```python
from build123d import *

# Parameters (mm, degrees)
SKETCH218_R     = 1.8
SKETCH218_R_2   = 1.5
PAD127054_DEPTH = 3
PAD127055_DEPTH = 2.5


with BuildPart() as base:
    # Sketch218 → Pad127054 (new body)
    with BuildSketch(Plane(origin=(50, 160, 11.5), x_dir=(1, 0, 0), z_dir=(0, 0, 1))):
        with BuildLine():
            Line((-40, 8.5), (-40, 10.5))
            Line((-40, 10.5), (-43, 10.5))
            Line((-43, 10.5), (-44.5, 10.5))
            Line((-44.5, 10.5), (-44.5, 7.5))
            Line((-44.5, 7.5), (-47.5, 7.5))
            Line((-47.5, 7.5), (-47.5, 10.5))
            Line((-47.5, 10.5), (-50, 10.5))
            Line((-50, -67), (-50, 10.5))
            Line((-28, -67), (-50, -67))
            Line((-24.376533, -53.477038), (-28, -67))
            Line((-29.344931, -44.194174), (-24.376533, -53.477038))
            Line((-22.98097, -37.830213), (-29.344931, -44.194174))
            Line((-22.98097, -37.830213), (-20.85965, -35.708892))
            Line((-20.85965, -35.708892), (-22.273864, -34.294679))
            Line((-17.847446, -29.868261), (-22.273864, -34.294679))
            Line((-24, -15.512303), (-17.847446, -29.868261))
            Line((-24, 0), (-24, -15.512303))
            ThreePointArc((-24, 0), (-24.87868, 2.12132), (-27, 3))
            Line((-37.721825, 3), (-27, 3))
            Line((-40, 8.5), (-37.721825, 3))
        make_face()
        with Locations((-27, 0)):
            Circle(SKETCH218_R, mode=Mode.SUBTRACT)
        with Locations((-27, -10)):
            Circle(SKETCH218_R, mode=Mode.SUBTRACT)
        with Locations((-23, -28)):
            Circle(SKETCH218_R, mode=Mode.SUBTRACT)
        with Locations((-35, 0)):
            Circle(SKETCH218_R, mode=Mode.SUBTRACT)
        with Locations((-32, -63)):
            Circle(SKETCH218_R_2, mode=Mode.SUBTRACT)
        with Locations((-42, -63)):
            Circle(SKETCH218_R_2, mode=Mode.SUBTRACT)
        with Locations((-32, -56)):
            Circle(SKETCH218_R_2, mode=Mode.SUBTRACT)
        with Locations((-42, -56)):
            Circle(SKETCH218_R_2, mode=Mode.SUBTRACT)
        with Locations((-44.4, -49)):
            Circle(SKETCH218_R, mode=Mode.SUBTRACT)
        with Locations((-44.4, -41)):
            Circle(SKETCH218_R, mode=Mode.SUBTRACT)
        with Locations((-44.4, -11)):
            Circle(SKETCH218_R, mode=Mode.SUBTRACT)
        with Locations((-44.4, -3)):
            Circle(SKETCH218_R, mode=Mode.SUBTRACT)
        with BuildLine():
            ThreePointArc((-43.5, -34), (-39, -38.5), (-34.5, -34))
            Line((-34.5, -34), (-34.5, -21))
            ThreePointArc((-34.5, -21), (-39, -16.5), (-43.5, -21))
            Line((-43.5, -34), (-43.5, -21))
        make_face(mode=Mode.SUBTRACT)
    extrude(amount=PAD127054_DEPTH)


with BuildPart() as base_mirror:
    # Part__Mirroring013: instance of Base
    add(base.part.mirror(Plane(origin=(0, 0, 0), x_dir=(0, -1, 0), z_dir=(1, 0, 0))))


with BuildPart() as mainfrontplate:
    # Sketch219 → Pad127055 (new body, symmetric)
    with BuildSketch(Plane(origin=(0, 0, 11.5), x_dir=(0, 1, 0), z_dir=(1, 0, 0))):
        Polygon((93, 0), (93, 5), (174.5, 5), (178, 1.5), (178, 0), align=None)
    extrude(amount=PAD127055_DEPTH, both=True)

    # Fusion004020030: union Base, Base (Mirror)
    add(base.part)
    add(base_mirror.part)


with BuildPart() as part_mirroring017:
    # Part__Mirroring017: instance of MainFrontPlate
    add(mainfrontplate.part.mirror(Plane(origin=(0, 0, 0), x_dir=(0, 1, 0), z_dir=(0, 0, 1))))


solid = part_mirroring017.part
```
Verification items for the finished model (mm, model axes). A direction names the side the tool comes from. Round coordinates to 2 decimals unless told otherwise and drop trailing zeros. Order: outer loops, then holes, each group sorted by start corner. A loop starts at its lowest first (then second) coordinate and runs counter-clockwise, first axis right, second up. Notation, with made-up numbers: (82.25, 60) -> (91.25, 60) arc R13 ccw to (91.25, 67) -> close; hole circle Ø4 at (-32.75, 35). An arc over 180 degrees is marked (long way). Put each result on its own line as item: value. Start each with the question number.
(1) Section check C-C (x = -11). Enter the section's corners in (y, z), then the cut area to 3 significant figures.
(2) Section check B-B (y = 157). Enter the section's corners in (x, z), then the cut area to 3 significant figures.
(3) Depth check by flat-ended pin: pin 1 Ø1.5 at (y, z) = (131.5, -13.5) entering from +X; pin 2 Ø3 at (y, z) = (114.5, -13.5) entering from -X; pin 3 Ø3 at (x, y) = (5.6, 157) entering from +Z; pin 4 Ø1.5 at (y, z) = (143.5, -14) entering from +X. Enter the tip coordinate at first touch or a pass-through.
(4) Section check A-A (x = 18). Enter the section's corners in (y, z).
(5) Tool access check on faces 4 (the face through (17.805, 98.487, -12.979)), 5 (the face through (18, 163, -13)), 6 (the face through (-8, 170.5, -13)), 7 (the face through (4, 167.5, -13)). Record the directions out of +Z, -Z, +X, -X, +Y, -Y that give a thin tool (end or side, any length) a straight path to the whole face; none if there is none.
(6) Section check D-D (y = 132). Enter the section's corners in (x, z).
(7) Draft check along X on faces 1 (the face through (23.84, 99.86, -12.98)), 2 (the face through (6.431, 109.403, -12.979)), 3 (the face through (-29.033, 137.41, -12.979)). Enter one of: +X half, -X half, draft (parallel to the pull), parting line (faces both ways), or undercut.
(8) Material ranges on line 1 along Y through (x, z) = (-5.6, -12.8); line 2 along X through (y, z) = (97, -13.5); line 3 along X through (y, z) = (104, -13.75), recorded low to high.
Completed:
1. outline: (93, -14.5) -> (121.5, -14.5) -> (121.5, -11.5) -> (93, -11.5) -> close; (143.5, -14.5) -> (166.09, -14.5) -> (166.09, -11.5) -> (143.5, -11.5) -> close
1. area: 153 mm2
2. outline: (-26, -14.5) -> (-7.4, -14.5) -> (-7.4, -11.5) -> (-26, -11.5) -> close; (-3.8, -14.5) -> (-2.5, -14.5) -> (-2.5, -16.5) -> (2.5, -16.5) -> (2.5, -14.5) -> (3.8, -14.5) -> (3.8, -11.5) -> (-3.8, -11.5) -> close; (7.4, -14.5) -> (26, -14.5) -> (26, -11.5) -> (7.4, -11.5) -> close
2. area: 144 mm2
3. pin 1: stops at x = 31.89
3. pin 2: stops at x = -22.16
3. pin 3: passes through
3. pin 4: stops at x = 26.74
4. outline: (93, -14.5) -> (95.5, -14.5) -> (95.5, -11.5) -> (93, -11.5) -> close; (98.5, -14.5) -> (102.5, -14.5) -> (102.5, -11.5) -> (98.5, -11.5) -> close; (105.5, -14.5) -> (163, -14.5) -> (163, -11.5) -> (105.5, -11.5) -> close
5. face 4: +Z, -Z
5. face 5: +Z, -Z, +X, +Y
5. face 6: +Z, -Z, -X, +Y
5. face 7: +Z, -Z, +Y
6. outline: (-31.35, -14.5) -> (-28.8, -14.5) -> (-28.8, -11.5) -> (-31.35, -11.5) -> close; (-25.2, -14.5) -> (-15.5, -14.5) -> (-15.5, -11.5) -> (-25.2, -11.5) -> close; (-6.5, -14.5) -> (-2.5, -14.5) -> (-2.5, -16.5) -> (2.5, -16.5) -> (2.5, -14.5) -> (6.5, -14.5) -> (6.5, -11.5) -> (-6.5, -11.5) -> close; (15.5, -14.5) -> (25.2, -14.5) -> (25.2, -11.5) -> (15.5, -11.5) -> close; (28.8, -14.5) -> (31.35, -14.5) -> (31.35, -11.5) -> (28.8, -11.5) -> close
7. face 1: +X half
7. face 2: undercut
7. face 3: -X half
8. line 1: y = 93 to 109.2, 112.8 to 117.2, 120.8 to 147.2, 150.8 to 155.2, 158.8 to 170.5
8. line 2: x = -23.07 to -19.5, -16.5 to -9.5, -6.5 to 6.5, 9.5 to 16.5, 19.5 to 23.07
8. line 3: x = -24.95 to -19.5, -16.5 to -9.5, -6.5 to 6.5, 9.5 to 16.5, 19.5 to 24.95
